The model under review builds one solid part; all positions refer to its coordinate system, in mm. Face numbers are marked on the shaded views. A direction names the side the tool comes from. Coordinates: 2 decimals unless noted, no trailing zeros. Write each loop counter-clockwise with the first axis right and the second up, starting at its lowest first coordinate (ties: lowest second). Pieces come first, ordered by that corner, then holes.
1) Add section B-B, the plane x = 22.5. State the section outline as (y, z) points.
2) Add section A-A, the plane y = -4. State the section outline as (x, z) points, then the cut area to 3 significant figures.
3) For line 1 (Z direction, x = 22.5, y = 10.45); line 2 (Y direction, x = 2.45, z = 3); line 3 (X direction, y = 11.4, z = 9), list the stretches that pass through material, from the lowest coordinate up.
4) Add section D-D, the plane x = 18.5. State the section outline as (y, z) points.
5) Add section C-C, the plane z = 3. State the section outline as (x, y) points, then the cut area to 3 significant figures.
6) Mouldability with a two-part tool opening along Y and no side actions: class the marked faces 1, 2, 3 and 4 as released by +Y, released by -Y, zero draft, split by the parting line, or undercut.
7) Machinability: for the marked faces 5 and 6, which of the approach directions +Z, -Z, +X, -X, +Y, -Y give a long, thin tool a straight path to every point of the face, cutting with its end or side? Answer none if there is none.
from build123d import *

# Parameters (mm, degrees)
SKETCH_1_W               = 34
SKETCH_1_H               = 26
SKETCH_1_W_2             = 26
SKETCH_1_H_2             = 15
EXTRUDE_1_DEPTH          = 25
SKETCH_2_R               = 1.5
CUT_EXTRUDE_1_DEPTH      = 45.158804332
SKETCH_3_R               = 2.5
CUT_EXTRUDE_2_DEPTH      = 4
CUT_EXTRUDE_4_DEPTH      = 47.917480751
CUT_EXTRUDE_4_DEPTH_BACK = 47.917480751
SKETCH_5_R               = 1.5
SKETCH_6_R               = 1.5
CUT_EXTRUDE_5_DEPTH      = 45.158804332


with BuildPart() as part:
    # 草图1 → 凸台-拉伸1 (new body)
    with BuildSketch(Plane.XY):
        with Locations((17, 0)):
            Rectangle(SKETCH_1_W, SKETCH_1_H)
        with Locations((17, 0)):
            Rectangle(SKETCH_1_W_2, SKETCH_1_H_2, mode=Mode.SUBTRACT)
    extrude(amount=EXTRUDE_1_DEPTH)

    # 草图2 → 切除-拉伸1 (cut, through all)
    with BuildSketch(Plane.XY.offset(25)):
        with Locations((5.5, 7.5)):
            Circle(SKETCH_2_R)
        with Locations((5.5, -7.5)):
            Circle(SKETCH_2_R)
        with Locations((28.5, -7.5)):
            Circle(SKETCH_2_R)
        with Locations((28.5, 7.5)):
            Circle(SKETCH_2_R)
    extrude(amount=-CUT_EXTRUDE_1_DEPTH, mode=Mode.SUBTRACT)

    # 草图3 → 切除-拉伸2 (cut)
    with BuildSketch(Plane.ZY):
        with Locations((10, 0)):
            Circle(SKETCH_3_R)
    extrude(amount=-CUT_EXTRUDE_2_DEPTH, mode=Mode.SUBTRACT)

    # 草图5 → 切除-拉伸4 (cut, two sides: drawn at the far end of the back side and taken through both)
    with BuildSketch(Plane(origin=(0, -7.5, 0), x_dir=(1, 0, 0), z_dir=(0, 1, 0)).offset(-CUT_EXTRUDE_4_DEPTH_BACK)):
        with Locations(Location((22.5, -22, 0), (0, 0, 270))):
            Circle(SKETCH_5_R)
        with Locations(Location((22.5, -9, 0), (0, 0, 270))):
            Circle(SKETCH_5_R)
    extrude(amount=CUT_EXTRUDE_4_DEPTH + CUT_EXTRUDE_4_DEPTH_BACK, mode=Mode.SUBTRACT)

    # 草图6 → 切除-拉伸5 (cut, through all)
    with BuildSketch(Plane(origin=(34, 0, 0), x_dir=(0, 0, -1), z_dir=(1, 0, 0))):
        with Locations((-3, 0)):
            Circle(SKETCH_6_R)
    extrude(amount=-CUT_EXTRUDE_5_DEPTH, mode=Mode.SUBTRACT)


solid = part.part
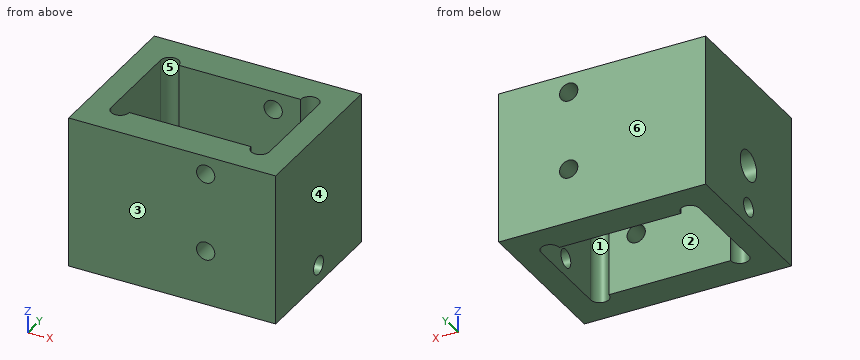
Geometry results:
1. outline: (-13, 0) - (-7.5, 0) - (-7.5, 7.5) - (-13, 7.5) - close; (-13, 10.5) - (-7.5, 10.5) - (-7.5, 20.5) - (-13, 20.5) - close; (-13, 23.5) - (-7.5, 23.5) - (-7.5, 25) - (-13, 25) - close; (7.5, 0) - (13, 0) - (13, 7.5) - (7.5, 7.5) - close; (7.5, 10.5) - (13, 10.5) - (13, 20.5) - (7.5, 20.5) - close; (7.5, 23.5) - (13, 23.5) - (13, 25) - (7.5, 25) - close
2. outline: (0, 0) - (4, 0) - (4, 25) - (0, 25) - close; (30, 0) - (34, 0) - (34, 25) - (30, 25) - close
2. area: 200 mm2
3. line 1: z = 0 to 7.5, 10.5 to 20.5, 23.5 to 25
3. line 2: y = -13 to -1.5, 1.5 to 13
3. line 3: x = 0 to 21, 24 to 34
4. outline: (-13, 0) - (-7.5, 0) - (-7.5, 25) - (-13, 25) - close; (7.5, 0) - (13, 0) - (13, 25) - (7.5, 25) - close
5. outline: (0, -13) - (34, -13) - (34, -1.5) - (30, -1.5) - (30, -7.5) arc R1.5 cw to (27, -7.5) - (7, -7.5) arc R1.5 cw to (4, -7.5) - (4, -1.5) - (0, -1.5) - close; (0, 1.5) - (4, 1.5) - (4, 7.5) arc R1.5 cw to (7, 7.5) - (27, 7.5) arc R1.5 cw to (30, 7.5) - (30, 1.5) - (34, 1.5) - (34, 13) - (0, 13) - close
5. area: 456 mm2
6. face 1: undercut
6. face 2: undercut
6. face 3: released by -Y
6. face 4: zero draft
7. face 5: +Z, -Z
7. face 6: +Z, -Z, +X, -X, +Y
